The model under review builds one solid part; all positions refer to its coordinate system, in mm. A direction names the side the tool comes from. Round coordinates to 2 decimals unless told otherwise and drop trailing zeros. Write each loop counter-clockwise with the first axis right and the second up, starting at its lowest first coordinate (ties: lowest second). Pieces come first, ordered by that corner, then holes. Notation, with made-up numbers: M -35,13 L -10,13 A6 ccw -10,19 Z; hole C 70,-15.75 d9. An arc over 180 degrees is marked long. One line per item, written item: value. Start each with the question number.
1) Take a section at C-C, the plane y = 23.75. Write out the cut boundary in (x, z), and give its area (3 significant figures).
2) Take a section at A-A, the plane x = 0. Write out the cut boundary in (y, z), and give its area (3 significant figures).
3) For P1, Ø1.5, axis at y = 6, z = -14, coming from the +X side; P2, Ø8, axis at x = 4.5, z = -10, coming from the -Y side; P3, Ø2.5, axis at x = -20, z = 2.5, coming from the -Y side; P4, Ø1.5, axis at x = -15, z = -14, coming from the -Y side, all flat-tipped, find the tip position at first contact; note any pin that passes through.
4) Mouldability with a two-part tool opening along X and no side actions: class faces 4 (the face through (-20.93, 18.18, -0.13)), 5 (the face through (-0.4, 19.3, -8.3)), 6 (the face through (20.17, 18.18, -4.66)) as +X half, -X half, draft (parallel to the pull), parting line (faces both ways), or undercut.
5) Tool access review of faces 1 (the face through (1.856, 23.572, 2.42)), 2 (the face through (-5.44, 16.258, -17.274)), 3 (the face through (-0.05, 21.14, 1.25)): name each direction out of +Z, -Z, +X, -X, +Y, -Y from which nothing blocks a thin tool from reaching the whole face with its end or side.
6) Take a section at B-B, the plane z = 0. State how many separate pieces and enclosed holes the cut face has, and give its area (3 significant figures).
7) Wall thickness on probe 1 along Y at (x, z) = (-1.5, 2); probe 2 along Y at (x, z) = (6.5, -11); probe 3 along Y at (x, z) = (-4, 1): over which ranges is each line inside the solid? List them lowest first.
8) Take a section at D-D, the plane x = 21.92. Write out the cut boundary in (y, z).
from build123d import *

# Parameters (mm, degrees)
BOSS_EXTRUDE1_START = -2.2
SKETCH2_R           = 1
BOSS_EXTRUDE1_DEPTH = 2.2


with BuildPart() as part:
    # Sketch1 → Revolve1 (revolve)
    with BuildSketch(Plane.XY, mode=Mode.PRIVATE) as revolve1_sk:
        Polygon((0, 25.6), (3.05, 25.6), (3.05, 21.6), (1.25, 21.6), (1.25, 20.7), (8, 20.7), (8, 19.3), (18.11, 19.3), (18.11, 13.3), (17.5, 13.3), (17.5, 6), (18.11, 6), (18.11, 0), (0, 0), align=None)
    revolve(revolve1_sk.sketch.rotate(Axis((0, 0, 0), (0, 1, 0)), 90), axis=Axis((0, 0, 0), (0, 1, 0)))

    # Sketch2 → Boss-Extrude1 (add)
    # profile 1 of 2: a face of its own
    with BuildSketch(Plane(origin=(0, 19.3, 0), x_dir=(1, 0, 0), z_dir=(0, 1, 0)).offset(BOSS_EXTRUDE1_START)):
        with BuildLine():
            Line((-23.3452514, 3.284061273), (-17.087191109, 6))
            ThreePointArc((-17.087191109, 6), (-18.11, 0), (-17.087191109, -6))
            Line((-17.087191109, -6), (-23.3452514, -3.284061273))
            ThreePointArc((-23.3452514, -3.284061273), (-25.5, 0), (-23.3452514, 3.284061273))
        make_face()
        with Locations(Location((-21.92, 0, 0), (0, 0, 270))):
            Circle(SKETCH2_R, mode=Mode.SUBTRACT)
    # profile 2 of 2: a face of its own
    with BuildSketch(Plane(origin=(0, 19.3, 0), x_dir=(1, 0, 0), z_dir=(0, 1, 0)).offset(BOSS_EXTRUDE1_START)):
        with BuildLine():
            Line((17.087191109, 6), (23.3452514, 3.284061273))
            ThreePointArc((23.3452514, 3.284061273), (25.5, 0), (23.3452514, -3.284061273))
            Line((23.3452514, -3.284061273), (17.087191109, -6))
            ThreePointArc((17.087191109, -6), (18.11, 0), (17.087191109, 6))
        make_face()
        with Locations(Location((21.92, 0, 0), (0, 0, 270))):
            Circle(SKETCH2_R, mode=Mode.SUBTRACT)
    extrude(amount=BOSS_EXTRUDE1_DEPTH)


solid = part.part
Checked values:
1. outline: C 0,0 d6.1
1. area: 29.2 mm2
2. outline: M 0,-18.11 L 6,-18.11 L 6,-17.5 L 13.3,-17.5 L 13.3,-18.11 L 19.3,-18.11 L 19.3,-8 L 20.7,-8 L 20.7,-1.25 L 21.6,-1.25 L 21.6,-3.05 L 25.6,-3.05 L 25.6,3.05 L 21.6,3.05 L 21.6,1.25 L 20.7,1.25 L 20.7,8 L 19.3,8 L 19.3,18.11 L 13.3,18.11 L 13.3,17.5 L 6,17.5 L 6,18.11 L 0,18.11 Z
2. area: 739 mm2
3. P1: stops at x = 12.35
3. P2: stops at y = 0
3. P3: stops at y = 17.1
3. P4: passes through
4. face 4: undercut
4. face 5: draft
4. face 6: +X half
5. face 1: +Y
5. face 2: -Y
5. face 3: none
6. separate pieces: 3
6. enclosed holes: 0
6. area: 763 mm2
7. probe 1: y = 0 to 20.7, 21.6 to 25.6
7. probe 2: y = 0 to 19.3
7. probe 3: y = 0 to 20.7
8. outline: M 17.1,-3.9 L 19.3,-3.9 L 19.3,-1 L 17.1,-1 Z; M 17.1,1 L 19.3,1 L 19.3,3.9 L 17.1,3.9 Z
